```python
from build123d import *

# Parameters (mm, degrees)
IZIM1_R                     = 1.5
Y_KSEKLIK_EKSTR_ZYON1_DEPTH = 5
KES_EKSTR_ZYON1_DEPTH       = 2.5
IZIM3_W                     = 40
IZIM3_H                     = 4.02
Y_KSEKLIK_EKSTR_ZYON7_DEPTH = 5


with BuildPart() as part:
    # Çizim1 → Yükseklik-Ekstrüzyon1 (new, symmetric)
    with BuildSketch(Plane.XY):
        with BuildLine():
            Line((-3, -1.02611879), (-3, -11.02611879))
            ThreePointArc((-3, -11.02611879), (0, -14.02611879), (3, -11.02611879))
            Line((3, -11.02611879), (3, -1.02611879))
            ThreePointArc((3, -1.02611879), (0, 1.97388121), (-3, -1.02611879))
        make_face()
        with Locations((0, -1.02611879)):
            Circle(IZIM1_R, mode=Mode.SUBTRACT)
        with Locations((0, -11.02611879)):
            Circle(IZIM1_R, mode=Mode.SUBTRACT)
    extrude(amount=Y_KSEKLIK_EKSTR_ZYON1_DEPTH, both=True)

    # Çizim2 → Kes-Ekstrüzyon1 (cut, symmetric)
    with BuildSketch(Plane.XY):
        with BuildLine():
            Line((-3, -1.02611879), (-3, -4.02611879))
            Line((-3, -4.02611879), (0, -4.02611879))
            Line((0, -4.02611879), (3, -4.02611879))
            Line((3, -4.02611879), (3, -1.02611879))
            ThreePointArc((3, -1.02611879), (0, 1.97388121), (-3, -1.02611879))
        make_face()
        with BuildLine():
            ThreePointArc((-3, -11.02611879), (0, -14.02611879), (3, -11.02611879))
            Line((3, -11.02611879), (3, -8.043702706))
            Line((3, -8.043702706), (-3, -8.043702706))
            Line((-3, -8.043702706), (-3, -11.02611879))
        make_face()
    extrude(amount=KES_EKSTR_ZYON1_DEPTH, both=True, mode=Mode.SUBTRACT)

    # Çizim3 → Yükseklik-Ekstrüzyon7 (add, symmetric)
    with BuildSketch(Plane.XY):
        with Locations((-23, -6.02611879)):
            Rectangle(IZIM3_W, IZIM3_H)
    extrude(amount=Y_KSEKLIK_EKSTR_ZYON7_DEPTH, both=True)


solid = part.part
```
Part model, mm, in its own coordinate system. A direction names the side the tool comes from. Round coordinates to 2 decimals unless told otherwise and drop trailing zeros. Write each loop counter-clockwise with the first axis right and the second up, starting at its lowest first coordinate (ties: lowest second). Pieces come first, ordered by that corner, then holes.
Item 1: Cut at D-D, the plane x = -9.5. Give the cut face in (y, z).
Results:
outline: (-8.04, -5) - (-4.02, -5) - (-4.02, 5) - (-8.04, 5) - close
Item 2: Cut at A-A, the plane x = 0. Give the cut face in (y, z), plus the area to 3 significant figures.
Results:
outline: (-14.03, -5) - (-12.53, -5) - (-12.53, -2.5) - (-14.03, -2.5) - close; (-14.03, 2.5) - (-12.53, 2.5) - (-12.53, 5) - (-14.03, 5) - close; (-9.53, -5) - (-2.53, -5) - (-2.53, -2.5) - (-4.03, -2.5) - (-4.03, 2.5) - (-2.53, 2.5) - (-2.53, 5) - (-9.53, 5) - (-9.53, 2.5) - (-8.04, 2.5) - (-8.04, -2.5) - (-9.53, -2.5) - close; (0.47, -5) - (1.97, -5) - (1.97, -2.5) - (0.47, -2.5) - close; (0.47, 2.5) - (1.97, 2.5) - (1.97, 5) - (0.47, 5) - close
area: 70.1 mm2
Item 3: Probe L1, parallel to Y at x = 0, z = -3.3; L2, parallel to Z at x = -1.5, y = -2; L3, parallel to Y at x = -35.5, z = -2. List the from-to ranges inside material, lowest first.
Results:
L1: y = -14.03 to -12.53, -9.53 to -2.53, 0.47 to 1.97
L2: z = -5 to -2.5, 2.5 to 5
L3: y = -8.04 to -4.02
Item 4: Drop flat-ended pins along their axis: pin 1 Ø3 at (x, y) = (-19.5, -1.5) entering from +Z; pin 2 Ø1.5 at (x, z) = (-5.5, 0.5) entering from +Y; pin 3 Ø1.5 at (x, z) = (1, 0.5) entering from -Y; pin 4 Ø1.2 at (y, z) = (-2, 3.5) entering from -X. Give the stop position or say it passes through.
Results:
pin 1: passes through
pin 2: stops at y = -4.02
pin 3: stops at y = -8.04
pin 4: stops at x = -3
Item 5: Which spindle directions (+Z, -Z, +X, -X, +Y, -Y) get a long thin tool onto all of the face, cutting with end or side? Do faces 4 (the flat face through (0, -8.044, 0)), 5 (the flat face through (-3, -10, 3)), 6 (the flat face through (-23, -4.016, 0)). Say none if no direction does.
Results:
face 4: +X, -X, -Y
face 5: +Z, -Z, -X, -Y
face 6: +Z, -Z, -X, +Y
Item 6: Two-plate mould, pull along X, no slides. Class faces 1 (the cylindrical face through (0.066, 1.973, -3.732)), 2 (the flat face through (-23, -8.036, 0)), 3 (the cylindrical face through (-1.5, -1, -3.8)): +X half, -X half, draft (parallel to the pull), parting line (faces both ways), or undercut.
Results:
face 1: parting line
face 2: draft
face 3: undercut
Item 7: Cut at B-B, the plane y = -8.5. Give the cut face in (x, z), plus the area to 3 significant figures.
Results:
outline: (-3, -5) - (3, -5) - (3, -2.5) - (-3, -2.5) - close; (-3, 2.5) - (3, 2.5) - (3, 5) - (-3, 5) - close
area: 30.0 mm2
